Can you work these out from the model? Positions are in its coordinate system, mm. A direction names the side the tool comes from. Coordinates: 2 decimals unless noted, no trailing zeros. Order: outer loops, then holes, each group sorted by start corner. A loop starts at its lowest first (then second) coordinate and runs counter-clockwise, first axis right, second up. Notation, with made-up numbers: (-4, 34) - (7, 34) arc R17 cw to (7, 42) - close; hole circle Ø2 at (-27, 8). An arc over 180 degrees is marked (long way). Return JSON: item names as keys, results as strings. Group by question number.
1) If I drill on line 1 along Y through (x, z) = (6.25, 0); line 2 along Z through (x, y) = (8, 0); line 3 along Z through (x, y) = (4.5, 0), over which ranges is the centre line in solid material (lowest first)?
2) For pin 1 Ø4 at (y, z) = (-6, 8) entering from +X; pin 2 Ø4 at (x, z) = (9.5, 0.5) entering from +Y; pin 3 Ø2 at (x, y) = (14, -2.5) entering from -Z, each with a flat end and sliding along its axis, tell me the tip position at first contact or that it passes through.
3) Imagine slicing it at A-A (z = 0). Write out the boundary of the cut face in (x, y), and give its area (3 significant figures).
4) Imagine slicing it at B-B (x = 16.5). Write out the boundary of the cut face in (y, z), and give its area (3 significant figures).
5) If we mould it in two halves opening along Y, with no side actions, what happens to faces 1 (the face through (2.465, -2.273, 9.666)), 2 (the face through (2.5, -9.1, -3.8)), 3 (the face through (5, 2, -5))? For each: pulls with the +Y half, pulls with the -Y half, needs draft (parallel to the pull), parting line crosses it, or undercut.
6) Which directions (+Z, -Z, +X, -X, +Y, -Y) give clear straight access to the entire face, cutting with the end or side of a thin tool? Please do faces 4 (the face through (2.465, -7.52, 6.484)), 5 (the face through (2.465, -0.825, -9.895)), 6 (the face through (2.46, 5.14, -7.08)), 7 (the face through (2.465, -0.814, 9.864)).
7) Imagine slicing it at C-C (z = -4). Write out the boundary of the cut face in (x, y).
```python
from build123d import *

# Parameters (mm, degrees)
BASPROSKE_W              = 5
BASPROSKE_H              = 11
TOOTHCUT_DEPTH           = 17.340134638
TEETHCUTS_COUNT          = 20
TEETHCUTS_ANGLE          = 342
BORSKE_R                 = 2.5
BORE_DEPTH               = 50.0000508
BOSS_EXTRUDE2_DEPTH      = 16
BOSS_EXTRUDE2_DEPTH_BACK = 5
SKETCH1_R                = 5
CUT_EXTRUDE1_DEPTH       = 27.061912983


with BuildPart() as part:
    # BasProSke → Base-Revolve (revolve)
    with BuildSketch(Plane(origin=(0, 0, 0), x_dir=(1, 0, 0), z_dir=(0, 1, 0)), mode=Mode.PRIVATE) as base_revolve_sk:
        with Locations((2.5, 5.5)):
            Rectangle(BASPROSKE_W, BASPROSKE_H)
    revolve(base_revolve_sk.sketch.rotate(Axis((-10, 0, 0), (1, 0, 0)), 180), axis=Axis((-10, 0, 0), (1, 0, 0)))

    # TooCutSke → ToothCut (cut, through all)
    with BuildSketch(Plane(origin=(0, 0, 0), x_dir=(0, 0, -1), z_dir=(1, 0, 0))):
        with BuildLine():
            ThreePointArc((0.589353609, 8.729127295), (0, 8.749), (-0.589353609, 8.729127295))
            ThreePointArc((-0.589353609, 8.729127295), (-0.82475631, 9.893403384), (-1.391689312, 10.937213814))
            ThreePointArc((-1.391689312, 10.937213814), (0, 11.0254), (1.391689312, 10.937213814))
            ThreePointArc((1.391689312, 10.937213814), (0.82475631, 9.893403384), (0.589353609, 8.729127295))
        make_face()
    toothcut = extrude(amount=TOOTHCUT_DEPTH, mode=Mode.SUBTRACT)

    # TeethCuts: ToothCut ×20 about axis
    teethcuts_axis = Axis((-10, 0, 0), (1, 0, 0))
    for i in range(1, TEETHCUTS_COUNT):
        add(toothcut.rotate(teethcuts_axis, i * TEETHCUTS_ANGLE / (TEETHCUTS_COUNT - 1)), mode=Mode.SUBTRACT)

    # BorSke → Bore (cut, symmetric)
    with BuildSketch(Plane(origin=(0, 0, 0), x_dir=(0, 0, -1), z_dir=(1, 0, 0))):
        with Locations(Location((0, 0, 0), (0, 0, 180))):
            Circle(BORSKE_R)
    extrude(amount=BORE_DEPTH, both=True, mode=Mode.SUBTRACT)

    # Sketch1 → Boss-Extrude2 (add, two sides: drawn at the far end of the back side and taken through both)
    with BuildSketch(Plane(origin=(5, 0, 0), x_dir=(0, 0, -1), z_dir=(1, 0, 0)).offset(-BOSS_EXTRUDE2_DEPTH_BACK)):
        Circle(SKETCH1_R)
    extrude(amount=BOSS_EXTRUDE2_DEPTH + BOSS_EXTRUDE2_DEPTH_BACK)

    # Sketch2 → Cut-Extrude1 (cut, through all)
    with BuildSketch(Plane(origin=(21, 0, 0), x_dir=(0, 0, -1), z_dir=(1, 0, 0))):
        with BuildLine():
            ThreePointArc((2.7, 0), (-1.132475165, 2.451020196), (-1.75, -2.056088519))
            Line((-1.75, -2.056088519), (1.75, -2.056088519))
            ThreePointArc((1.75, -2.056088519), (2.451020196, -1.132475165), (2.7, 0))
        make_face()
    extrude(amount=-CUT_EXTRUDE1_DEPTH, mode=Mode.SUBTRACT)


solid = part.part
```
Calculated:
{
 "1": {"line 1": "-5 to -2.06, 2.7 to 5", "line 2": "-5 to -2.7, 2.7 to 5", "line 3": "-8.75 to -2.7, 2.7 to 8.75"},
 "2": {"pin 1": "x = 5", "pin 2": "y = 5", "pin 3": "z = -4.77"},
 "3": {"outline": "(0, -8.75) - (5, -8.75) - (5, -5) - (21, -5) - (21, -2.06) - (0, -2.06) - close; (0, 2.7) - (21, 2.7) - (21, 5) - (5, 5) - (5, 8.75) - (0, 8.75) - close", "area": "148 mm2"},
 "4": {"outline": "circle Ø10 at (0, 0); hole (-2.06, -1.75) arc R2.7 ccw (long way) to (-2.06, 1.75) - close", "area": "57.2 mm2"},
 "5": {"face 1": "undercut", "face 2": "pulls with the -Y half", "face 3": "needs draft"},
 "6": {"face 4": "+X, -X, -Y", "face 5": "-Z, +X, -X", "face 6": "+X, -X", "face 7": "+Z, +X, -X"},
 "7": {"outline": "(0, -9.34) - (5, -9.34) - (5, -3) - (21, -3) - (21, 3) - (5, 3) - (5, 9.34) - (0, 9.34) - close"}
}
